Input: dimensioned drawing with shaded views. Units: mm. Origin: part minimum x, y, z. A direction names the side the tool comes from. Coordinates: 2 decimals unless noted, no trailing zeros. Order: outer loops, then holes, each group sorted by start corner. A loop starts at its lowest first (then second) coordinate and runs counter-clockwise, first axis right, second up. Notation, with made-up numbers: (-38.75, 69) -> (-20.75, 69) arc R35 cw to (-20.75, 103) -> close; hole circle Ø5 at (-11.75, 81). An arc over 180 degrees is marked (long way). Put each result on its own line as item: value.
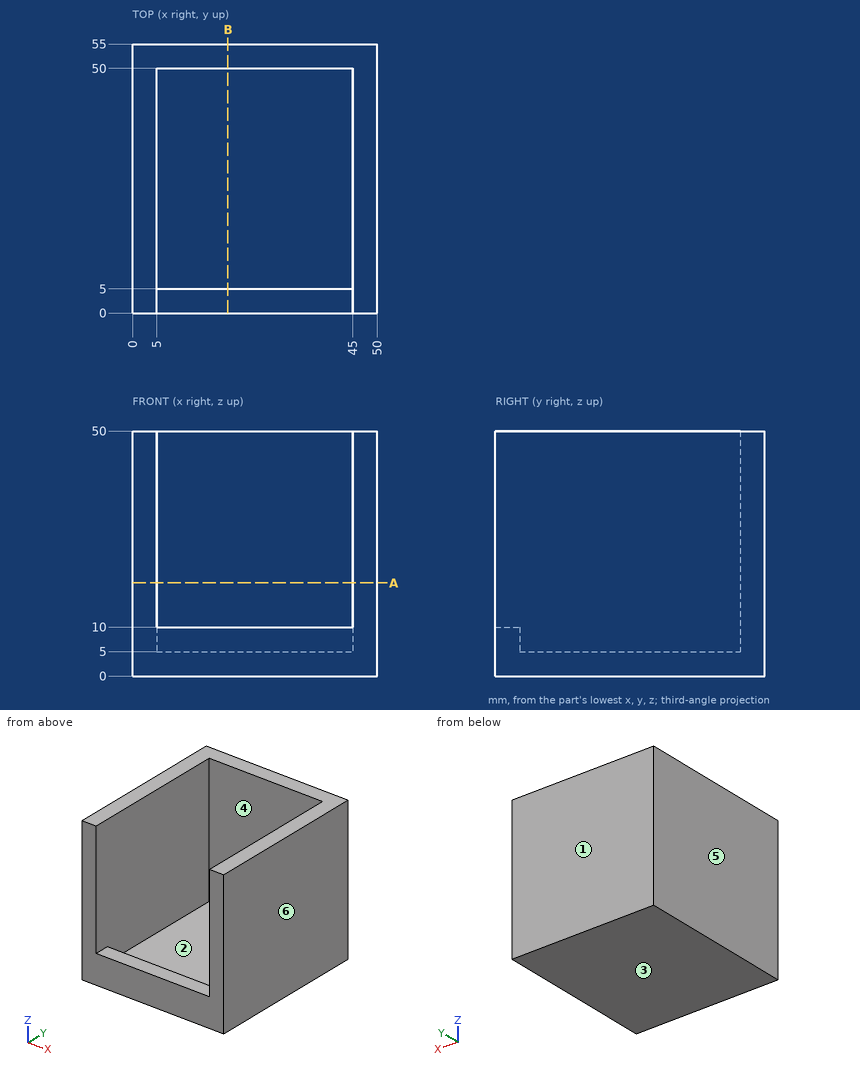
1. Cut plane B-B on x = 19.5. Output: boundary loops of the cut face in (y, z), plus the area to 3 significant figures.
Numbers:
outline: (0, 0) -> (55, 0) -> (55, 50) -> (50, 50) -> (50, 5) -> (5, 5) -> (5, 10) -> (0, 10) -> close
area: 525 mm2
2. Ray query, line 1 along X through (y, z) = (18, 8); line 2 along Z through (x, y) = (28.5, 32); line 3 along Y through (x, z) = (25.5, 22). Return the intervals inside material, ascending.
Numbers:
line 1: x = 0 to 5, 45 to 50
line 2: z = 0 to 5
line 3: y = 50 to 55
3. Set-up query: the marked faces 1 and 2. Return all of +Z, -Z, +X, -X, +Y, -Y with unobstructed straight access to the full face (end or side cutting, diameter ignored); none if empty.
Numbers:
face 1: +Z, -Z, +X, -X, +Y
face 2: +Z
4. Cut plane A-A on z = 19. Output: boundary loops of the cut face in (x, y), plus the area to 3 significant figures.
Numbers:
outline: (0, 0) -> (5, 0) -> (5, 50) -> (45, 50) -> (45, 0) -> (50, 0) -> (50, 55) -> (0, 55) -> close
area: 750 mm2
5. Pull-direction query (X, two-part tool) for the marked faces 3, 4, 5 and 6; classes: pulls with the +X half, pulls with the -X half, needs draft (parallel to the pull), parting line crosses it, or undercut.
Numbers:
face 3: needs draft
face 4: undercut
face 5: pulls with the -X half
face 6: pulls with the +X half
6. First-contact query: pin 1 (5 mm diameter, centred on x = 32, y = 30.5, fed in from +Z); pin 2 (2 mm diameter, centred on x = 24.5, z = 34, fed in from -Y); pin 3 (1.5 mm diameter, centred on x = 28.5, y = 2, fed in from +Z). Flat tips, straight axial feed; report the tip coordinate or a pass-through.
Numbers:
pin 1: stops at z = 5
pin 2: stops at y = 50
pin 3: stops at z = 10
